from build123d import *

# Parameters (mm, degrees)
F1_DEPTH = 2.5
F0_R     = 6.5
F2_DEPTH = 5


with BuildPart() as f1:
    # F0 (on Top) → F1 (new body)
    with BuildSketch(Plane.XY):
        with BuildLine():
            ThreePointArc((-29.64832, 11.779182), (-23.637873, 9.289611), (-21.148259, 3.279182))
            ThreePointArc((-21.148259, 3.279182), (-21.185854, 2.480628), (-21.298304, 1.689138))
            Line((-21.298304, 1.689138), (31.998499, 1.689138))
            ThreePointArc((31.998499, 1.689138), (33.799692, 8.698623), (40.3483, 11.77968))
            Line((40.3483, 11.77968), (-29.64832, 11.779182))
        make_face()
    extrude(amount=F1_DEPTH)

    # F0 (on Top) → F2 (join)
    with BuildSketch(Plane.XY):
        with BuildLine():
            ThreePointArc((-21.298304, 1.689138), (-21.185854, 2.480628), (-21.148259, 3.279182))
            ThreePointArc((-21.148259, 3.279182), (-23.637873, 9.289611), (-29.64832, 11.779182))
            ThreePointArc((-29.64832, 11.779182), (-36.196728, -2.140003), (-21.298304, 1.689138))
        make_face()
        with Locations((-29.648259, 3.279182)):
            Circle(F0_R, mode=Mode.SUBTRACT)
        with BuildLine():
            ThreePointArc((48.84836, 3.27968), (46.358747, 9.290109), (40.3483, 11.77968))
            ThreePointArc((40.3483, 11.77968), (33.799692, 8.698623), (31.998499, 1.689138))
            ThreePointArc((31.998499, 1.689138), (41.147167, -5.182702), (48.84836, 3.27968))
        make_face()
        with Locations((40.34836, 3.27968)):
            Circle(F0_R, mode=Mode.SUBTRACT)
    extrude(amount=F2_DEPTH)


solid = f1.part
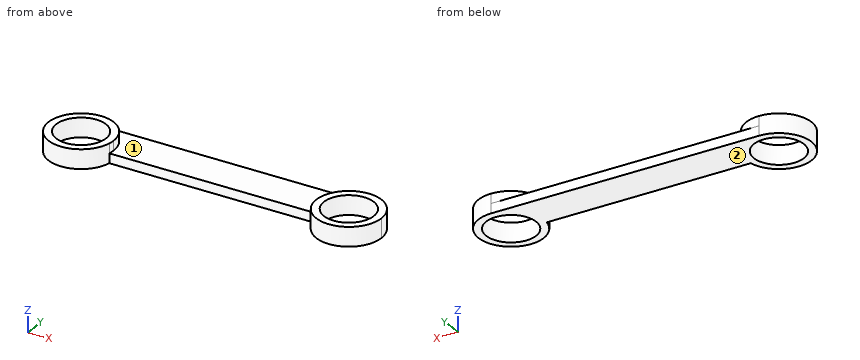
Work out the finished part from the listing and answer in its coordinate system (mm). Face numbers are marked on the shaded views. Give positions to 0.01 mm unless a question says otherwise; leave off trailing zeros. Order: outer loops, then holes, each group sorted by start corner. A loop starts at its lowest first (then second) coordinate and runs counter-clockwise, first axis right, second up. Notation, with made-up numbers: (33.5, -35.75) -> (85.5, -35.75) arc R19 cw to (85.5, -25.75) -> close; hole circle Ø7 at (25.25, 72.5). An arc over 180 degrees is marked (long way). Answer as a JSON object with one key per item and string values. Group by question number.
1. Section D-D on y = 4 is taken. Determine the outline of the cut face in (x, z), plus the area to 3 significant figures.
2. Section A-A on z = 3.7 is taken. Determine the outline of the cut face in (x, y), plus the area to 3 significant figures.
3. Section C-C on y = 0.5 is taken. Determine the outline of the cut face in (x, z), plus the area to 3 significant figures.
4. The mould has two halves that part along X. Classify the marked faces 1 and 2: released by +X, released by -X, zero draft, split by the parting line, or undercut.
5. Section B-B on x = -31.5 is taken. Determine the outline of the cut face in (y, z).
6. Flat-ended cylindrical pins translate along their axes: pin 1 Ø3 at (x, z) = (2.5, 1.5) entering from -Y; pin 2 Ø1.5 at (y, z) = (5.5, 4) entering from +X; pin 3 Ø8 at (x, y) = (-5.5, 6) entering from +Z; pin 4 Ø8 at (x, y) = (-29.65, 3.28) entering from -Z. Find the tip coordinate at first contact, or state that the pin passes through.
7. Consider line 1 along X through (y, z) = (6.25, 3.8); line 2 along X through (y, z) = (5, 3.6); line 3 along X through (y, z) = (7.25, 0.55). Determine where each line is inside the solid, lowest interval first. Write a range as [from, to].
Result sheet:
{
 "1": {"outline": "(-38.12, 0) -> (-36.11, 0) -> (-36.11, 5) -> (-38.12, 5) -> close; (-23.19, 0) -> (33.89, 0) -> (33.89, 5) -> (31.88, 5) -> (31.88, 2.5) -> (-21.18, 2.5) -> (-21.18, 5) -> (-23.19, 5) -> close; (46.81, 0) -> (48.82, 0) -> (48.82, 5) -> (46.81, 5) -> close", "area": "173 mm^2"},
 "2": {"outline": "(-21.3, 1.69) arc R8.5 ccw to (-21.15, 3.28) arc R8.5 ccw (long way) to start; (40.35, 11.78) arc R8.5 ccw (long way) to (48.85, 3.28) arc R8.5 ccw to start; hole circle Ø13 at (-29.65, 3.28); hole circle Ø13 at (40.35, 3.28)", "area": "188 mm^2"},
 "3": {"outline": "(-37.68, 0) -> (-35.52, 0) -> (-35.52, 5) -> (-37.68, 5) -> close; (-23.77, 0) -> (-21.62, 0) -> (-21.62, 5) -> (-23.77, 5) -> close; (32.32, 0) -> (34.47, 0) -> (34.47, 5) -> (32.32, 5) -> close; (46.22, 0) -> (48.38, 0) -> (48.38, 5) -> (46.22, 5) -> close", "area": "43.1 mm^2"},
 "4": {"face 1": "undercut", "face 2": "zero draft"},
 "5": {"outline": "(-5.02, 0) -> (-2.95, 0) -> (-2.95, 5) -> (-5.02, 5) -> close; (9.51, 0) -> (11.58, 0) -> (11.58, 5) -> (9.51, 5) -> close"},
 "6": {"pin 1": "stops at y = 1.69", "pin 2": "stops at x = 48.72", "pin 3": "stops at z = 2.5", "pin 4": "passes through"},
 "7": {"line 1": "x = [-37.61, -35.43], [-23.87, -21.68], [32.38, 34.57], [46.13, 48.31]", "line 2": "x = [-37.97, -35.92], [-23.38, -21.32], [32.02, 34.08], [46.62, 48.67]", "line 3": "x = [-37.16, -34.79], [-24.5, 35.2], [45.49, 47.86]"}
}
